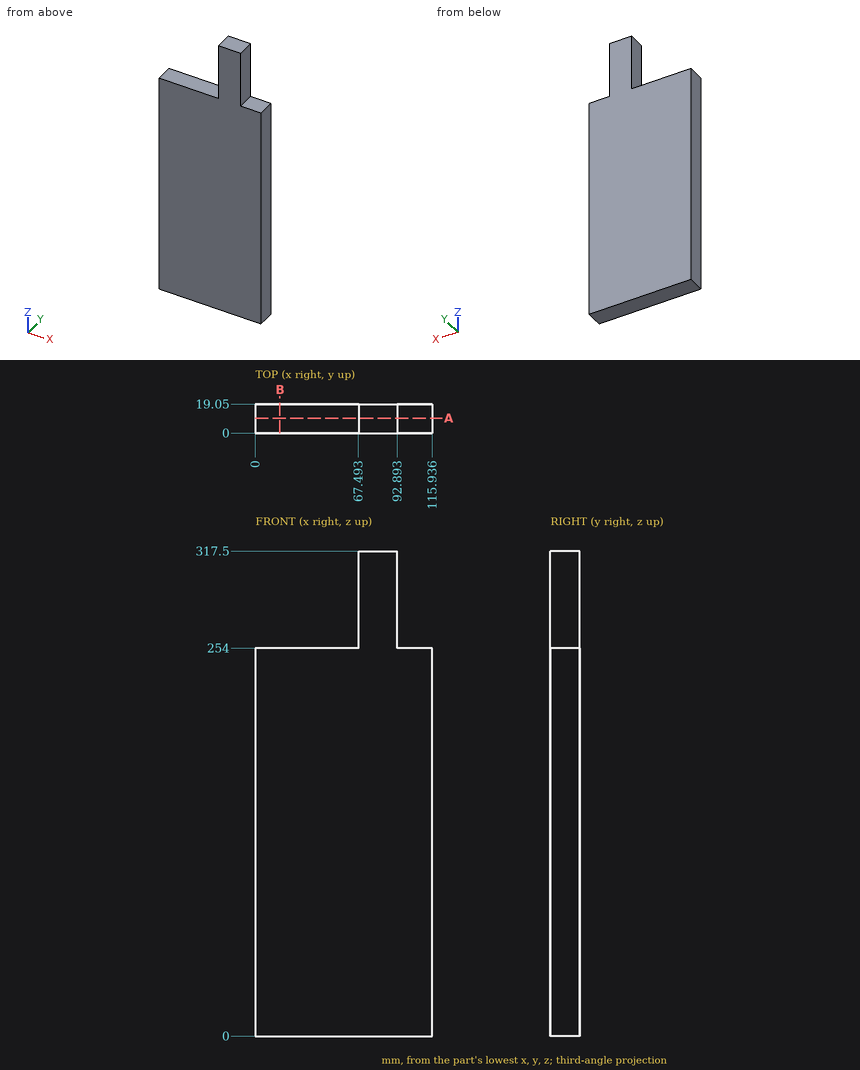
For this review, use the dimensioned drawing (mm, ordinates from the lowest corner) and the shaded views. Give positions to 0.01 mm unless a question says otherwise; leave off trailing zeros. Order: outer loops, then holes, each group sorted by start corner. A loop starts at its lowest first (then second) coordinate and runs counter-clockwise, first axis right, second up. Notation, with made-up numbers: M -28,-30.5 L 17,-30.5 A25 cw 17,-0.5 Z; hole C -21,-35.75 d2. An arc over 180 degrees is marked long. One line per question, with ' | ' between items. Start each with the question number.
1) Wall thickness on L1, parallel to Z at x = 99, y = 1.75; L2, parallel to X at y = 7.5, z = 282.5: over which ranges is each line inside the solid? List them lowest first. Write a range as from..to.
2) Consider section A-A, the plane y = 9.75. Give the boundary of the cut face in (x, z), then the cut area to 3 significant figures.
3) Clearance check with a flat-ended pin moving along its axis: P1, Ø1, axis at x = 24, y = 9.5, coming from the +Z side. State where the tip first meets the part, or that it passes through.
4) Consider section B-B, the plane x = 16. Give the boundary of the cut face in (y, z).
Found:
1) L1: z = 0..254 | L2: x = 67.49..92.89
2) outline: M 0,0 L 115.94,0 L 115.94,254 L 92.89,254 L 92.89,317.5 L 67.49,317.5 L 67.49,254 L 0,254 Z | area: 31,100 mm²
3) P1: stops at z = 254
4) outline: M 0,0 L 19.05,0 L 19.05,254 L 0,254 Z
